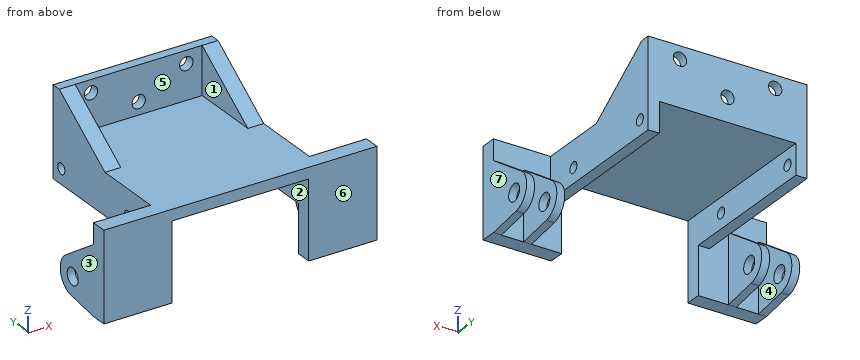
from build123d import *

# Parameters (mm, degrees)
SKETCH_1_W               = 50
SKETCH_1_H               = 40
EXTRUDE_1_DEPTH          = 5
SKETCH_2_W               = 6
SKETCH_2_H               = 40
EXTRUDE_2_DEPTH          = 8
SKETCH_4_W               = 38
SKETCH_4_H               = 40
CUT_EXTRUDE_2_DEPTH      = 1.5
SKETCH_6_R               = 1.7
CUT_EXTRUDE_3_DEPTH      = 45
CUT_EXTRUDE_3_DEPTH_BACK = 7
SKETCH_7_W               = 43
SKETCH_7_H               = 9.5
CUT_EXTRUDE_4_DEPTH      = 41
SKETCH_8_W               = 50
SKETCH_8_H               = 3
EXTRUDE_4_DEPTH          = 15
SKETCH_9_R               = 2.1
CUT_EXTRUDE_5_DEPTH      = 4
EXTRUDE_5_DEPTH          = 12
SKETCH_11_W              = 13
SKETCH_11_H              = 5
EXTRUDE_6_DEPTH          = 18
SKETCH_12_W              = 13
SKETCH_12_H              = 5
EXTRUDE_7_DEPTH          = 18
SKETCH_13_W              = 21.5
SKETCH_13_H              = 5
EXTRUDE_8_DEPTH          = 15
EXTRUDE_11_DEPTH         = 5
EXTRUDE_12_DEPTH         = 5
SKETCH_20_R              = 2.65
EXTRUDE_13_DEPTH         = 12
SKETCH_21_W              = 7
SKETCH_21_H              = 34.173261611
CUT_EXTRUDE_8_DEPTH      = 44


with BuildPart() as part:
    # 草图1 → 凸台-拉伸1 (new body)
    with BuildSketch(Plane.XY):
        Rectangle(SKETCH_1_W, SKETCH_1_H)
    extrude(amount=EXTRUDE_1_DEPTH)

    # 草图2 → 凸台-拉伸2 (add)
    with BuildSketch(Plane(origin=(0, 0, 0), x_dir=(-1, 0, 0), z_dir=(0, 0, -1))):
        with Locations((-22, 0)):
            Rectangle(SKETCH_2_W, SKETCH_2_H)
        with Locations((22, 0)):
            Rectangle(SKETCH_2_W, SKETCH_2_H)
    extrude(amount=EXTRUDE_2_DEPTH)

    # 草图4 → 切除-拉伸2 (cut)
    with BuildSketch(Plane(origin=(0, 0, 0), x_dir=(-1, 0, 0), z_dir=(0, 0, -1))):
        Rectangle(SKETCH_4_W, SKETCH_4_H)
    extrude(amount=-CUT_EXTRUDE_2_DEPTH, mode=Mode.SUBTRACT)

    # 草图6 → 切除-拉伸3 (cut, two sides)
    with BuildSketch(Plane(origin=(-19, 0, 0), x_dir=(0, 0, -1), z_dir=(1, 0, 0))) as cut_extrude_3_sk:
        with Locations((3.25, 16)):
            Circle(SKETCH_6_R)
        with Locations((3.25, -16)):
            Circle(SKETCH_6_R)
    extrude(amount=CUT_EXTRUDE_3_DEPTH, mode=Mode.SUBTRACT)
    extrude(cut_extrude_3_sk.sketch, amount=-CUT_EXTRUDE_3_DEPTH_BACK, mode=Mode.SUBTRACT)

    # 草图7 → 切除-拉伸4 (cut, through all)
    with BuildSketch(Plane.XZ.offset(20)):
        with Locations((0, -3.25)):
            Rectangle(SKETCH_7_W, SKETCH_7_H)
    extrude(amount=-CUT_EXTRUDE_4_DEPTH, mode=Mode.SUBTRACT)

    # 草图8 → 凸台-拉伸4 (add)
    with BuildSketch(Plane.XY.offset(5)):
        with Locations((0, 18.5)):
            Rectangle(SKETCH_8_W, SKETCH_8_H)
    extrude(amount=EXTRUDE_4_DEPTH)

    # 草图9 → 切除-拉伸5 (cut, through all)
    with BuildSketch(Plane.XZ.offset(-17)):
        with Locations((-15, 16)):
            Circle(SKETCH_9_R)
        with Locations((15, 16)):
            Circle(SKETCH_9_R)
        with Locations((0, 9)):
            Circle(SKETCH_9_R)
    extrude(amount=-CUT_EXTRUDE_5_DEPTH, mode=Mode.SUBTRACT)

    # 草图10 → 凸台-拉伸5 (add)
    with BuildSketch(Plane.XZ.offset(20)):
        Polygon((-25, -8), (-21.5, -8), (-21.5, 1.5), (21.5, 1.5), (21.5, -8), (25, -8), (25, 5), (-25, 5), align=None)
    extrude(amount=EXTRUDE_5_DEPTH)

    # 草图11 → 凸台-拉伸6 (add)
    with BuildSketch(Plane(origin=(25, 0, 0), x_dir=(0, 0, -1), z_dir=(1, 0, 0))):
        with Locations((1.5, -29.5)):
            Rectangle(SKETCH_11_W, SKETCH_11_H)
    extrude(amount=EXTRUDE_6_DEPTH)

    # 草图12 → 凸台-拉伸7 (add)
    with BuildSketch(Plane.ZY.offset(25)):
        with Locations((-1.5, -29.5)):
            Rectangle(SKETCH_12_W, SKETCH_12_H)
    extrude(amount=EXTRUDE_7_DEPTH)

    # 草图13 → 凸台-拉伸8 (add)
    with BuildSketch(Plane(origin=(0, 0, -8), x_dir=(-1, 0, 0), z_dir=(0, 0, -1))):
        with Locations((32.25, -29.5)):
            Rectangle(SKETCH_13_W, SKETCH_13_H)
        with Locations((-32.25, -29.5)):
            Rectangle(SKETCH_13_W, SKETCH_13_H)
    extrude(amount=EXTRUDE_8_DEPTH)

    # 草图18 → 凸台-拉伸11 (add)
    with BuildSketch(Plane.ZY.offset(25)):
        Polygon((5, -5), (20, 17), (5, 17), align=None)
    extrude(amount=-EXTRUDE_11_DEPTH)

    # 草图19 → 凸台-拉伸12 (add)
    with BuildSketch(Plane(origin=(25, 0, 0), x_dir=(0, 0, -1), z_dir=(1, 0, 0))):
        Polygon((-5, 17), (-5, -5), (-20, 17), align=None)
    extrude(amount=-EXTRUDE_12_DEPTH)

    # 草图20 → 凸台-拉伸13 (add)
    with BuildSketch(Plane.ZY.offset(43)):
        with BuildLine():
            Line((-23, -27), (-21.438888742, -16.145833443))
            ThreePointArc((-21.438888742, -16.145833443), (-16.842939484, -11.152221487), (-10.528814426, -13.640340197))
            Line((-10.528814426, -13.640340197), (-1.5, -27))
            Line((-1.5, -27), (-23, -27))
        make_face()
        with Locations((-15.5, -17)):
            Circle(SKETCH_20_R, mode=Mode.SUBTRACT)
    extrude_13 = extrude(amount=-EXTRUDE_13_DEPTH)

    # 草图21 → 切除-拉伸8 (cut, through all)
    with BuildSketch(Plane(origin=(0, 0, -23), x_dir=(-1, 0, 0), z_dir=(0, 0, -1))):
        with Locations((37, -9.913369194)):
            Rectangle(SKETCH_21_W, SKETCH_21_H)
    cut_extrude_8 = extrude(amount=-CUT_EXTRUDE_8_DEPTH, mode=Mode.SUBTRACT)

    # 镜向3: 凸台-拉伸13, 切除-拉伸8 across plane
    add(extrude_13.mirror(Plane(origin=(0, 0, 0), x_dir=(0, 0, 1), z_dir=(1, 0, 0))))
    add(cut_extrude_8.mirror(Plane(origin=(0, 0, 0), x_dir=(0, 0, 1), z_dir=(1, 0, 0))), mode=Mode.SUBTRACT)


solid = part.part
Source: CAD feature listing. Evaluate the final solid. Frame: model axes, mm. Face numbers are marked on the shaded views. A direction names the side the tool comes from. Coordinates: 2 decimals unless noted, no trailing zeros. Order: outer loops, then holes, each group sorted by start corner. A loop starts at its lowest first (then second) coordinate and runs counter-clockwise, first axis right, second up.
Item 1: Cut plane D-D (y = -22.5). Return loops of the section in (x, z), plus the area to 3 significant figures.
Output values:
outline: (-43, -22.35) - (-40.5, -22.35) - (-40.5, -4.54) - (-43, -4.54) - close; (-33.5, -22.35) - (-31, -22.35) - (-31, -4.54) - (-33.5, -4.54) - close; (-25, -8) - (-21.5, -8) - (-21.5, 1.5) - (21.5, 1.5) - (21.5, -8) - (25, -8) - (25, 5) - (-25, 5) - close; (31, -22.35) - (33.5, -22.35) - (33.5, -4.54) - (31, -4.54) - close; (40.5, -22.35) - (43, -22.35) - (43, -4.54) - (40.5, -4.54) - close
area: 420 mm2
Item 2: Cut plane A-A (x = 15). Return loops of the section in (y, z).
Output values:
outline: (-32, 1.5) - (20, 1.5) - (20, 13.9) - (17, 13.9) - (17, 5) - (-32, 5) - close; (17, 18.1) - (20, 18.1) - (20, 20) - (17, 20) - close
Item 3: Cut plane B-B (z = 9). Return loops of the section in (x, y), plus the area to 3 significant figures.
Output values:
outline: (-25, 0.87) - (-20, 0.87) - (-20, 17) - (-2.1, 17) - (-2.1, 20) - (-25, 20) - close; (2.1, 17) - (20, 17) - (20, 0.87) - (25, 0.87) - (25, 20) - (2.1, 20) - close
area: 299 mm2
Item 4: First-contact query: P1, Ø4, axis at x = 23.5, y = -5.5, coming from the -Z side; P2, Ø12, axis at y = 7, z = 15.5, coming from the +X side; P3, Ø4, axis at y = -16, z = -3.25, coming from the -X side. Flat tips, straight axial feed; report the tip coordinate or a pass-through.
Output values:
P1: stops at z = -8
P2: stops at x = 25
P3: stops at x = -25
Item 5: Material intervals for line 1 (Y direction, x = 23.15, z = -3.25); line 2 (X direction, y = -12.5, z = -13.5); line 3 (Z direction, x = -15, y = 18.05), sorted ascending.
Output values:
line 1: y = -32 to -17.7, -14.3 to 14.3, 17.7 to 20
line 2: x = -43 to -40.5, -33.5 to -31, 31 to 33.5, 40.5 to 43
line 3: z = 1.5 to 13.9, 18.1 to 20
Item 6: Set-up query: the marked faces 1, 2, 3 and 4. Return all of +Z, -Z, +X, -X, +Y, -Y with unobstructed straight access to the full face (end or side cutting, diameter ignored); none if empty.
Output values:
face 1: +Z, -Y
face 2: -Z, +Y, -Y
face 3: +Z, -Z, -X, +Y, -Y
face 4: +Z, -Z, +Y
Item 7: Cut plane C-C (y = -9). Return loops of the section in (x, z), plus the area to 4 significant figures.
Output values:
outline: (-25, -8) - (-21.5, -8) - (-21.5, 1.5) - (21.5, 1.5) - (21.5, -8) - (25, -8) - (25, 5) - (-25, 5) - close
area: 241.5 mm2
Item 8: Pull-direction query (X, two-part tool) for the marked faces 5, 6 and 7; classes: pulls with the +X half, pulls with the -X half, needs draft (parallel to the pull), parting line crosses it, or undercut.
Output values:
face 5: undercut
face 6: needs draft
face 7: pulls with the +X half
